Geometry: see drawing. Coordinates: mm, zero at the bounding-box minimum. Coordinates: 2 decimals unless noted, no trailing zeros. Loops run counter-clockwise (first coordinate to the right, second up) from the corner with the lowest first, then second, coordinate; pieces in that order, holes last. Notation, with made-up numbers: (68.25, 73.25) -> (109.25, 73.25) arc R17 ccw to (109.25, 89.25) -> close; hole circle Ø2 at (25.5, -12). An arc over 180 degrees is marked (long way). One line per item, written item: value. Start each with the question number.
Item 1: Section query B-B on y = 23. Return loops of the section in (x, z).
Item 2: Section query A-A on z = 0.65. Return loops of the section in (x, y), then the cut area to 3 significant figures.
Item 3: Ray query, probe 1 along X at (y, z) = (15, 1.1); probe 2 along Y at (x, z) = (8, 0.9). Return the intervals inside material, ascending. Write a range as from..to.
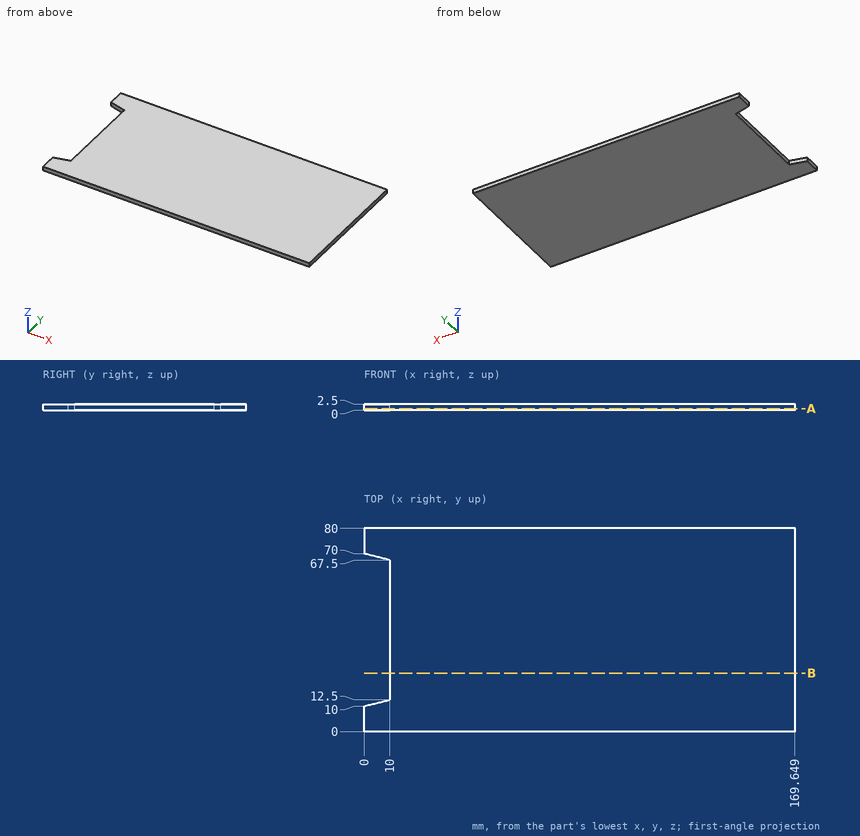
Reply:
1. outline: (10, 0) -> (169.65, 0) -> (169.65, 2.5) -> (10, 2.5) -> close
2. outline: (0, 0) -> (169.65, 0) -> (169.65, 80) -> (0, 80) -> (0, 70) -> (10, 67.5) -> (10, 12.5) -> (0, 10) -> close
2. area: 13,000 mm²
3. probe 1: x = 10..169.65
3. probe 2: y = 0..12, 68..80
